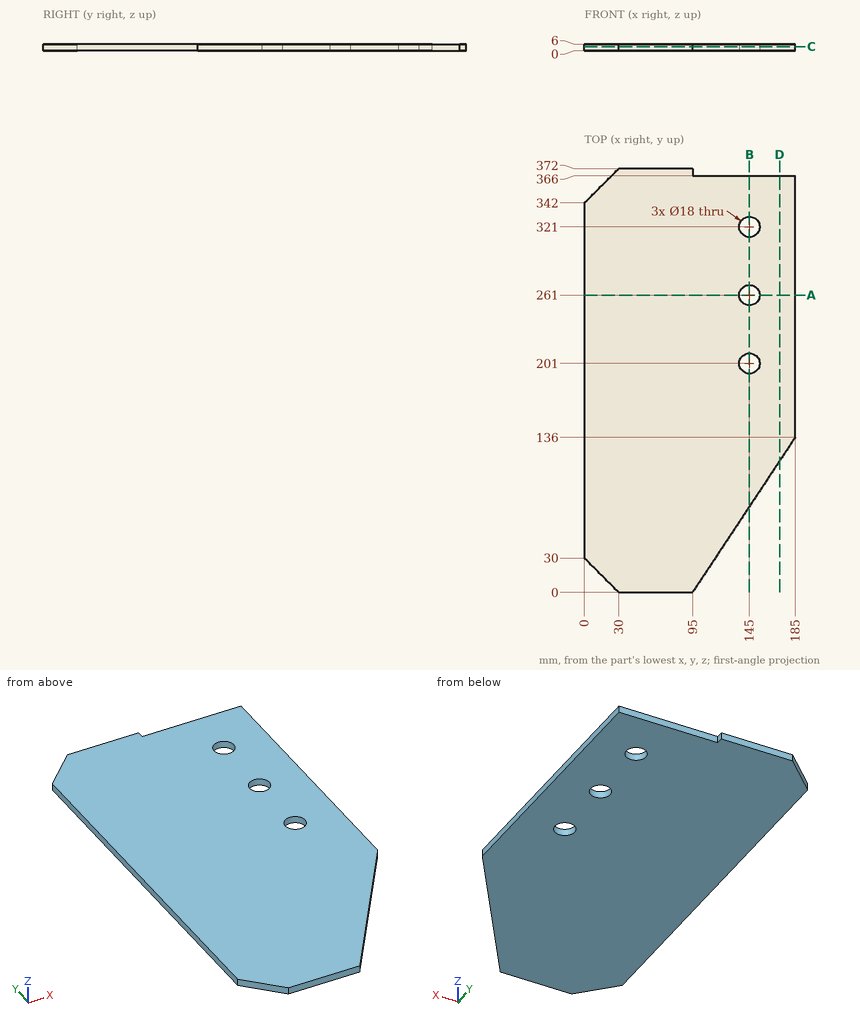
Job drawing, mm, ordinate dimensions from the low corner. One solid piece. Coordinates: 2 decimals unless noted, no trailing zeros. Write each loop counter-clockwise with the first axis right and the second up, starting at its lowest first coordinate (ties: lowest second). Pieces come first, ordered by that corner, then holes. Notation, with made-up numbers: (63, -4) - (67, -4) arc R11 ccw to (67, 15) - close; hole circle Ø3 at (52.5, 48). An arc over 180 degrees is marked (long way). Use a Markdown table: item, result. Add a question column.
Item 1: Band-saw the part on B-B, the plane x = 145. Give the cut face in (y, z), and give its area (3 significant figures).
Item 2: Band-saw the part on D-D, the plane x = 171.5. Give the cut face in (y, z), and give its area (3 significant figures).
Item 3: Band-saw the part on A-A, the plane y = 261. Give the cut face in (x, z), and give its area (3 significant figures).
Item 4: Flat gauge pins, fed straight in: pin 1 (1.8 mm diameter, centred on x = 149, z = 3.5, fed in from +Y); pin 2 (3 mm diameter, centred on y = 368.5, z = 4, fed in from +X). Where does each tip first touch, or does it go through?
Item 5: Band-saw the part on C-C, the plane z = 3.8. Give the cut face in (x, y), and give its area (3 significant figures).
Item 6: Drill centre lines: L1, parallel to X at y = 201, z = 1.7; L2, parallel to Y at x = 145, z = 4.25; L3, parallel to X at y = 96, z = 3.35. Where is each one in solid material? Low to high. Write a range as from..to.
Numbers:
| question | item | result |
|---|---|---|
| 1 | outline | (75.56, 0) - (192, 0) - (192, 6) - (75.56, 6) - close; (210, 0) - (252, 0) - (252, 6) - (210, 6) - close; (270, 0) - (312, 0) - (312, 6) - (270, 6) - close; (330, 0) - (366, 0) - (366, 6) - (330, 6) - close |
| 1 | area | 1,420 mm2 |
| 2 | outline | (115.6, 0) - (366, 0) - (366, 6) - (115.6, 6) - close |
| 2 | area | 1,500 mm2 |
| 3 | outline | (0, 0) - (136, 0) - (136, 6) - (0, 6) - close; (154, 0) - (185, 0) - (185, 6) - (154, 6) - close |
| 3 | area | 1,000 mm2 |
| 4 | pin 1 | y = 366 |
| 4 | pin 2 | x = 95 |
| 5 | outline | (0, 30) - (30, 0) - (95, 0) - (185, 136) - (185, 366) - (95, 366) - (95, 372) - (30, 372) - (0, 342) - close; hole circle Ø18 at (145, 201); hole circle Ø18 at (145, 261); hole circle Ø18 at (145, 321) |
| 5 | area | 60,500 mm2 |
| 6 | L1 | 0..136, 154..185 |
| 6 | L2 | 75.56..192, 210..252, 270..312, 330..366 |
| 6 | L3 | 0..158.53 |
